Could you check a few things on this model? Use its own coordinates, in mm. A direction names the side the tool comes from. Round coordinates to 2 decimals unless told otherwise and drop trailing zeros. One line per item, written item: value. Start each with the question number.
Q1. Please list where these lines run through material, in increasing order: line 1 along Z through (x, y) = (11.5, -45.5); line 2 along X through (y, z) = (-44, 12.25); line 3 along Y through (x, z) = (51, 16).
Q2. Thinking about a two-plate mould opening in X: for faces 3 (the face through (-320, 1, 19)), 4 (the face through (-5, 65, 10)), 5 (the face through (340, -1, 10)), which applies, released by +X, released by -X, zero draft, split by the parting line, or undercut?
Q3. Which directions (+Z, -Z, +X, -X, +Y, -Y) give clear straight access to the entire face, cutting with the end or side of a thin tool? Please do faces 1 (the face through (-5, -65, 5)), 2 (the face through (7, -50, 10)).
Q4. I'm going to push flat-ended pins straight in: pin 1 Ø9 at (x, y) = (-14.5, -47.5) entering from +Z; pin 2 Ø8 at (x, y) = (-322.5, 25.5) entering from +Z. Where does each tip first touch, or does it pass through?
from build123d import *

# Parameters (mm, degrees)
CROQUIS1_W              = 680
CROQUIS1_H              = 130
SALIENTE_EXTRUIR1_DEPTH = 20
CORTAR_EXTRUIR6_DEPTH   = 10
REDONDEO6_R             = 3
REDONDEO7_R             = 3
CORTAR_EXTRUIR9_DEPTH   = 1
CORTAR_EXTRUIR10_DEPTH  = 1


with BuildPart() as part:
    # Croquis1 → Saliente-Extruir1 (new body)
    with BuildSketch(Plane.XY):
        Rectangle(CROQUIS1_W, CROQUIS1_H)
    extrude(amount=SALIENTE_EXTRUIR1_DEPTH)

    # Croquis4 → Cortar-Extruir6 (cut)
    with BuildSketch(Plane.XY.offset(20)):
        with BuildLine():
            Line((-87.688515054, -65), (104.950033766, -65))
            ThreePointArc((104.950033766, -65), (8.630759356, -31.56754978), (-87.688515054, -65))
        make_face()
    extrude(amount=-CORTAR_EXTRUIR6_DEPTH, mode=Mode.SUBTRACT)

    # Redondeo6
    redondeo6_edges = [part.edges().sort_by_distance(p)[0] for p in [
        (8.630759356, -31.56754978, 20),
    ]]
    fillet(redondeo6_edges, radius=REDONDEO6_R)

    # Redondeo7
    redondeo7_edges = [part.edges().sort_by_distance(p)[0] for p in [
        (8.630759356, -65, 10),
    ]]
    fillet(redondeo7_edges, radius=REDONDEO7_R)

    # Croquis5 → Cortar-Extruir9 (cut)
    with BuildSketch(Plane.XY.offset(20)):
        Polygon((310, 65), (310, -65), (330, -65), (330, -5), (337, -5), (337, 15), (330, 15), (330, 65), align=None)
    extrude(amount=-CORTAR_EXTRUIR9_DEPTH, mode=Mode.SUBTRACT)

    # Croquis6 → Cortar-Extruir10 (cut)
    with BuildSketch(Plane.XY.offset(20)):
        Polygon((-310, 65), (-310, -65), (-330, -65), (-330, -5), (-337, -5), (-337, 15), (-330, 15), (-330, 65), align=None)
    extrude(amount=-CORTAR_EXTRUIR10_DEPTH, mode=Mode.SUBTRACT)


solid = part.part
Report:
1. line 1: z = 0 to 10
1. line 2: x = -340 to -52.29, 69.55 to 340
1. line 3: y = -37.45 to 65
2. face 3: undercut
2. face 4: zero draft
2. face 5: released by +X
3. face 1: +Z, -Z, +X, -X, -Y
3. face 2: +Z, -Y
4. pin 1: stops at z = 10
4. pin 2: stops at z = 19
